Can you work these out from the model? Positions are in its coordinate system, mm. Face numbers are marked on the shaded views. Round coordinates to 2 decimals unless told otherwise and drop trailing zeros. Loops run counter-clockwise (first coordinate to the right, second up) from the corner with the lowest first, then second, coordinate; pieces in that order, holes last. Notation, with made-up numbers: (7.5, -11) - (47.5, -11) arc R36 ccw to (47.5, 25) - close; hole circle Ø6 at (-16, 29.25). An arc over 180 degrees is marked (long way). Answer as CSV lines item,"result".
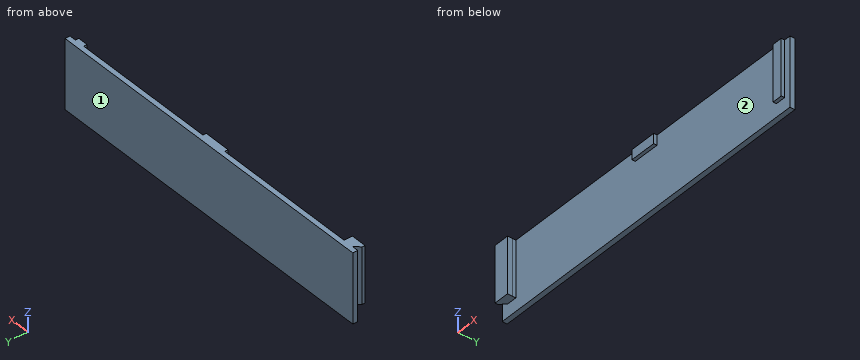
```python
from build123d import *

# Parameters (mm, degrees)
SKETCH026_W   = 106
SKETCH026_H   = 21
PAD_DEPTH     = 1.5
SKETCH027_W   = 3
SKETCH027_H   = 17
SKETCH027_W_2 = 8
SKETCH027_H_2 = 3
PAD012_DEPTH  = 1
PAD014_DEPTH  = 17


with BuildPart() as part:
    # Sketch026 → Pad (new body)
    with BuildSketch(Plane.XZ.offset(-104)):
        with Locations((-96, 16.5)):
            Rectangle(SKETCH026_W, SKETCH026_H)
    extrude(amount=PAD_DEPTH)

    # Sketch027 (on Face6 of Pad) → Pad012 (join)
    with BuildSketch(Plane.XZ.offset(-102.5)):
        with Locations((-145.5, 18.5)):
            Rectangle(SKETCH027_W, SKETCH027_H)
        with Locations((-46.5, 18.5)):
            Rectangle(SKETCH027_W, SKETCH027_H)
        with Locations((-96, 25.5)):
            Rectangle(SKETCH027_W_2, SKETCH027_H_2)
    extrude(amount=PAD012_DEPTH)

    # Sketch030 (on Face13 of Pad012) → Pad014 (join)
    with BuildSketch(Plane(origin=(0, 0, 10), x_dir=(1, 0, 0), z_dir=(0, 0, -1))):
        Polygon((-147.000002, -102.500002), (-148.600002, -100.900002), (-148.600002, -100.000001), (-144, -100), (-144.000002, -102.500002), align=None)
    extrude(amount=-PAD014_DEPTH)


with BuildPart() as part_1:
    # Body011 placement: moved
    add(part.part.moved(Location((192, 0, 0))))


solid = part_1.part
```
Q1. Imagine slicing it at B-B (x = 79.5). Write out the boundary of the cut face in (y, z).
Checks:
outline,"(102.5, 6) - (104, 6) - (104, 27) - (102.5, 27) - close"
Q2. I'm going to push flat-ended pins straight in: pin 1 Ø0.8 at (y, z) = (102, 15.5) entering from +X; pin 2 Ø8 at (x, z) = (61, 12) entering from -Y; pin 3 Ø2.5 at (x, z) = (97.5, 26) entering from -Y. Where does each tip first touch, or does it pass through?
Checks:
pin 1,"x = 147"
pin 2,"y = 102.5"
pin 3,"y = 101.5"
Q3. If I drill on line 1 along Y through (x, z) = (141, 24.5); line 2 along X through (y, z) = (100.45, 14.5); line 3 along X through (y, z) = (101.7, 10.5), over which ranges is the centre line in solid material (lowest first)? Write a range as [from, to].
Checks:
line 1,"[102.5, 104]"
line 2,"[43.4, 48]"
line 3,"[44.2, 48], [144, 147]"
Q4. We'd pull the mould along X, two halves only. Please class the marked faces 1 and 2: pulls with the +X half, pulls with the -X half, needs draft (parallel to the pull), parting line crosses it, or undercut.
Checks:
face 1,"needs draft"
face 2,"undercut"
